Part model, mm, in its own coordinate system. Give positions to 0.01 mm unless a question says otherwise; leave off trailing zeros. Order: outer loops, then holes, each group sorted by start corner. A loop starts at its lowest first (then second) coordinate and runs counter-clockwise, first axis right, second up. Notation, with made-up numbers: (8.25, 86) - (47.25, 86) arc R17 ccw to (47.25, 95) - close; hole circle Ø11 at (-13.75, 38.25). An arc over 180 degrees is marked (long way). One line per item, written item: value.
```python
from build123d import *

# Parameters (mm, degrees)
SKETCH1_R           = 7.5
SKETCH1_R_2         = 5
BOSS_EXTRUDE1_DEPTH = 2
BOSS_EXTRUDE2_DEPTH = 2
FILLET1_R           = 10
SKETCH4_R           = 11
SKETCH4_R_2         = 2
CUT_EXTRUDE1_DEPTH  = 2
SKETCH6_R           = 6.8
CUT_EXTRUDE2_DEPTH  = 10
SKETCH8_R           = 1.5
CUT_EXTRUDE3_DEPTH  = 179.433043373
SKETCH9_R           = 1.5
CUT_EXTRUDE4_DEPTH  = 10


with BuildPart() as part:
    # Sketch1 → Boss-Extrude1 (new body)
    with BuildSketch(Plane(origin=(0, 0, 0), x_dir=(1, 0, 0), z_dir=(0, 1, 0))):
        Polygon((0, 76.188021535), (-65.980762114, -38.094010768), (65.980762114, -38.094010768), align=None)
        with Locations(Location((0, 46.188021535, 0), (0, 0, 270))):
            Circle(SKETCH1_R, mode=Mode.SUBTRACT)
        with Locations(Location((-40, -23.094010768, 0), (0, 0, 270))):
            Circle(SKETCH1_R, mode=Mode.SUBTRACT)
        with Locations(Location((40, -23.094010768, 0), (0, 0, 270))):
            Circle(SKETCH1_R, mode=Mode.SUBTRACT)
        with Locations(Location((0, 0, 0), (0, 0, 270))):
            Circle(SKETCH1_R_2, mode=Mode.SUBTRACT)
    extrude(amount=BOSS_EXTRUDE1_DEPTH)

    # Sketch2 → Boss-Extrude2 (add)
    with BuildSketch(Plane(origin=(0, 2, 0), x_dir=(1, 0, 0), z_dir=(0, 1, 0))):
        Polygon((43.490381057, 0.860471904), (22.490381057, 37.233538863), (132.394191624, 100.686533479), (153.394191624, 64.313466521), align=None)
    extrude(amount=-BOSS_EXTRUDE2_DEPTH)

    # Fillet1
    fillet1_edges = [part.edges().sort_by_distance(p)[0] for p in [
        (153.394191624, 1, -64.313466521),
        (43.490381057, 1, -0.860471904),
        (22.490381057, 1, -37.233538863),
        (132.394191624, 1, -100.686533479),
        (65.980762114, 1, 38.094010768),
        (-65.980762114, 1, 38.094010768),
        (0, 1, -76.188021535),
    ]]
    fillet(fillet1_edges, radius=FILLET1_R)

    # Sketch4 → Cut-Extrude1 (cut)
    with BuildSketch(Plane(origin=(0, 2, 0), x_dir=(1, 0, 0), z_dir=(0, 1, 0))):
        with Locations(Location((33.774990748, 19.5, 0), (0, 0, 270))):
            Circle(SKETCH4_R)
        with Locations(Location((39.448384506, 40.673393759, 0), (0, 0, 270))):
            Circle(SKETCH4_R_2)
        with Locations(Location((54.948384506, 13.826606241, 0), (0, 0, 270))):
            Circle(SKETCH4_R_2)
        with Locations(Location((28.101596989, -1.673393759, 0), (0, 0, 270))):
            Circle(SKETCH4_R_2)
        with Locations(Location((12.601596989, 25.173393759, 0), (0, 0, 270))):
            Circle(SKETCH4_R_2)
    extrude(amount=-CUT_EXTRUDE1_DEPTH, mode=Mode.SUBTRACT)

    # Sketch6 → Cut-Extrude2 (cut)
    with BuildSketch(Plane(origin=(0, 2, 0), x_dir=(1, 0, 0), z_dir=(0, 1, 0))):
        with Locations(Location((129.903810568, 75, 0), (0, 0, 270))):
            Circle(SKETCH6_R)
    extrude(amount=-CUT_EXTRUDE2_DEPTH, mode=Mode.SUBTRACT)

    # Sketch8 → Cut-Extrude3 (cut, through all)
    with BuildSketch(Plane(origin=(0, 2, 0), x_dir=(1, 0, 0), z_dir=(0, 1, 0))):
        with Locations(Location((133.564064606, 88.660254038, 0), (0, 0, 270))):
            Circle(SKETCH8_R)
        with Locations(Location((143.564064606, 71.339745962, 0), (0, 0, 270))):
            Circle(SKETCH8_R)
        with Locations(Location((126.24355653, 61.339745962, 0), (0, 0, 270))):
            Circle(SKETCH8_R)
        with Locations(Location((116.24355653, 78.660254038, 0), (0, 0, 270))):
            Circle(SKETCH8_R)
    extrude(amount=-CUT_EXTRUDE3_DEPTH, mode=Mode.SUBTRACT)

    # Sketch9 → Cut-Extrude4 (cut)
    with BuildSketch(Plane(origin=(0, 2, 0), x_dir=(1, 0, 0), z_dir=(0, 1, 0))):
        with Locations(Location((57.201905284, 50.923393759, 0), (0, 0, 270))):
            Circle(SKETCH9_R)
        with Locations(Location((72.701905284, 24.076606241, 0), (0, 0, 270))):
            Circle(SKETCH9_R)
        with Locations(Location((111.673048454, 46.576606241, 0), (0, 0, 270))):
            Circle(SKETCH9_R)
        with Locations(Location((96.173048454, 73.423393759, 0), (0, 0, 270))):
            Circle(SKETCH9_R)
    extrude(amount=-CUT_EXTRUDE4_DEPTH, mode=Mode.SUBTRACT)


solid = part.part
```
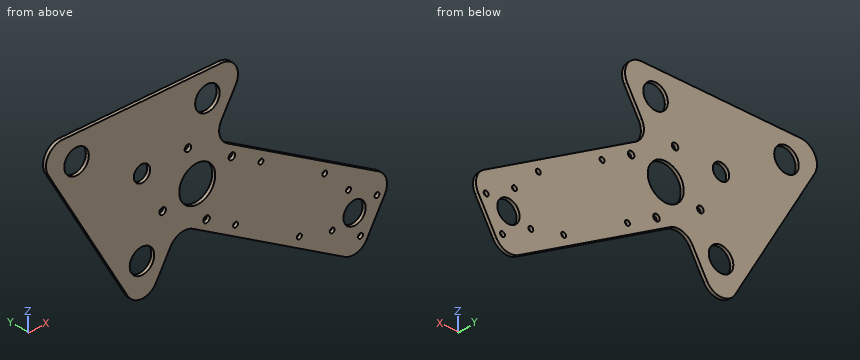
1) Slice it at C-C on y = 1.5. Count the separate pieces of the cut face and the enclosed holes in it, then the cut area to 3 significant figures.
Answer:
separate pieces: 1
enclosed holes: 18
area: 11,400 mm2
2) Slice it at A-A on x = 0. Write the cut outline in (y, z), then the cut area to 3 significant figures.
Answer:
outline: (0, -66.19) - (2, -66.19) - (2, -53.69) - (0, -53.69) - close; (0, -38.69) - (2, -38.69) - (2, -5) - (0, -5) - close; (0, 5) - (2, 5) - (2, 38.09) - (0, 38.09) - close
area: 159 mm2
3) Slice it at D-D on x = 89. Write the cut outline in (y, z).
Answer:
outline: (0, -75.63) - (2, -75.63) - (2, -27.14) - (0, -27.14) - close
4) Drop a flat-ended pin along its axis: P1, Ø1.8, axis at x = 111.67, z = -46.58, coming from the +Y side. Give the stop position or say it passes through.
Answer:
P1: passes through
5) Wall check: line 1 along Z through (x, y) = (125, 1.55); line 2 along X through (y, z) = (1.75, 22.5); line 3 along X through (y, z) = (1.35, -51). Give the ranges that are in metal, low to high. Write a range as [from, to].
Answer:
line 1: z = [-96.3, -79.71], [-70.29, -62.18], [-60.5, -47.92]
line 2: x = [-56.98, -47.48], [-32.52, 32.52], [47.48, 56.98]
line 3: x = [-14.54, -5.75], [5.75, 14.54], [46.33, 55.7], [58.7, 130.33]
6) Slice it at B-B on z = -19.5. Write the cut outline in (x, y) (3 decimals), then the cut area to 3 significant figures.
Answer:
outline: (-32.729, 0) - (22.775, 0) - (22.775, 2) - (-32.729, 2) - close; (44.775, 0) - (75.775, 0) - (75.775, 2) - (44.775, 2) - close
area: 173 mm2
